Work out the finished part from the listing and answer in its coordinate system (mm). A direction names the side the tool comes from. Give positions to 0.01 mm unless a question says otherwise; leave off trailing zeros. Loops run counter-clockwise (first coordinate to the right, second up) from the corner with the lowest first, then second, coordinate; pieces in that order, holes last. Notation, with made-up numbers: M -9,-35.75 L 19,-35.75 A20 cw 19,-0.75 Z; hole C -13.75,52 d11. An arc over 180 degrees is marked long. Write item = value, one per line. Start each with the question number.
1. Section C-C on x = -25.5 is taken. Determine the outline of the cut face in (y, z) (3 decimals).
2. The mould has two halves that part along Y. Classify faces 1 (the face through (7.2, -39.1, 3.7)), 2 (the face through (14, -39, 2)), 3 (the face through (-20.855, -58.623, 23.909)): released by +Y, released by -Y, zero draft, split by the parting line, or undercut.
3. Consider L1, parallel to Y at x = 9, z = 2.15 (3 decimals); L2, parallel to X at y = -39.5, z = 3; L3, parallel to Z at x = -28, y = -44.25. Determine where each line is inside the solid, lowest interval first. Write a range as [from, to].
4. Section A-A on x = 9 is taken. Determine the outline of the cut face in (y, z) (3 decimals), plus the area to 3 significant figures.
5. Flat-ended cylindrical pins translate along their axes: pin 1 Ø2 at (y, z) = (-55, 27) entering from -X; pin 2 Ø5 at (x, z) = (-25, 22.5) entering from +Y (3 decimals); pin 3 Ø1.5 at (y, z) = (-40.5, 17.5) entering from -X; pin 4 Ø8 at (y, z) = (-44.5, 4.5) entering from +X. Find the tip coordinate at first contact, or state that the pin passes through.
6. For faces 4 (the face through (12, -38, 5)), 5 (the face through (-20, -55, 27)), 6 (the face through (-39.1, -35.38, 29.02)), 7 (the face through (-30, -55, 27)), determine the directions among +Z, -Z, +X, -X, +Y, -Y from which every point of the face is accessible in a straight line to the end or side of a thin tool.
7. Section B-B on z = 24 is taken. Determine the outline of the cut face in (x, y) (3 decimals).
8. Section D-D on z = 3 is taken. Determine the outline of the cut face in (x, y) (3 decimals), plus the area to 3 significant figures.
Autodesk Inventor part; units mm, degrees
ref_plane "РабПлоскость1" through (0, 0, 0) normal (0, 0, 1) x (1, 0, 0)
ref_plane "YZ Plane" through (0, 0, 0) normal (1, 0, 0) x (0, 1, 0)
ref_plane "XZ Plane" through (0, 0, 0) normal (0, 1, 0) x (-1, 0, 0)
ref_plane "РабПлоскость1" through (0, 0, 0) normal (0, 0, 1) x (1, 0, 0)
sketch "Эскиз1" plane through (0, 0, 0) normal (0, 0, 1) x (1, 0, 0)
  line L0 (-6, -50.525) -> (-6, 46.475)
  arc A0 (-10, -54.525) -> (-6, -50.525) centre (-10, -50.525) ccw
  line L1 (-36, -54.525) -> (-10, -54.525)
  arc A1 (-40, -50.525) -> (-36, -54.525) centre (-36, -50.525) ccw
  line L2 (-40, 46.475) -> (-40, -50.525)
  circle A2 centre (-1, -39.525) radius 5
  line L3 (5, 13.475) -> (5, 17.5589)
  line L4 (14, -44.525) -> (4, -44.525)
  line L5 (4, -44.525) -> (4, -34.525)
  line L6 (4, -34.525) -> (14, -34.525)
  line L7 (14, -34.525) -> (14, -44.525)
  line L8 (4, -44.525) -> (-1, -44.525)
  line L9 (-1, -44.525) -> (-1, -34.525)
  line L10 (-1, -34.525) -> (4, -34.525)
  line L11 (4, -34.525) -> (4, -44.525)
  point P0 (0, 0)
  dimension "d0" = 10
  dimension "d1" = 10
  dimension "d2" = 5
  dimension "d3" = 10
  dimension "d4" = 15
  dimension "d5" = 20
extrude "Выдавливание1" add sketch "Эскиз1" along normal blind 5
sketch "Эскиз2" plane through (0, 0, 5) normal (0, 0, 1) x (1, 0, 0)
  line L0 (-1, -44.525) -> (14, -44.525)
  line L1 (14, -44.525) -> (14, -34.525)
  line L2 (14, -34.525) -> (-1, -34.525)
  arc A0 (-1, -34.525) -> (-1, -44.525) centre (-1, -39.525) ccw
  circle A1 centre (-1, -39.525) radius 5
  line L3 (-1, -44.525) -> (4, -44.525)
  line L4 (4, -44.525) -> (4, -34.525)
  line L5 (4, -34.525) -> (-1, -34.525)
  line L6 (-1, -34.525) -> (-1, -44.525)
  point P0 (0, 0)
  point P1 (4, -44.525)
  dimension "d8" = 10
extrude "Выдавливание2" add sketch "Эскиз2" along normal blind 22.5 contours A1 L4 L0 | L6 A1 | A0 L6 | L2 L4 A1
sketch "Эскиз3" plane through (0, 0, 27.5) normal (0, 0, 1) x (1, 0, 0)
  line L0 (-1, -44.525) -> (4, -44.525)
  line L1 (4, -44.525) -> (4, -34.525)
  line L2 (4, -34.525) -> (-1, -34.525)
  arc A0 (-1, -34.525) -> (-1, -44.525) centre (-1, -39.525) ccw
  line L3 (4, -34.525) -> (-40, -34.525)
  line L4 (-40, -34.525) -> (-40, -44.525)
  line L5 (-40, -44.525) -> (4, -44.525)
  line L6 (4, -44.525) -> (4, -34.525)
  line L7 (-40, 46.475) -> (-40, -50.525)
  line L8 (-30, -34.525) -> (-20, -34.525)
  line L9 (-20, -34.525) -> (-20, -59.525)
  line L10 (-20, -59.525) -> (-30, -59.525)
  line L11 (-30, -59.525) -> (-30, -34.525)
  line L12 (-36, -54.525) -> (-10, -54.525)
  point P0 (0, 0)
  point P1 (-1, -34.525)
  point P2 (-20, -44.525)
  point P3 (-30, -44.525)
  dimension "d11" = 0
  dimension "d12" = 10
  dimension "d24" = 10
  dimension "d25" = 10
  dimension "d26" = 5
extrude "Выдавливание3" add sketch "Эскиз3" along normal blind 3
sketch "Эскиз4" plane through (0, 0, 5) normal (0, 0, 1) x (1, 0, 0)
  line L0 (4, -34.525) -> (4, -44.525)
  line L1 (4, -44.525) -> (14, -44.525)
  line L2 (14, -44.525) -> (14, -34.525)
  line L3 (14, -34.525) -> (4, -34.525)
  circle A0 centre (9, -39.525) radius 1.6899
  point P0 (0, 0)
hole "Отверстие1" at (9, -39.525, 5) direction (0, 0, -1) diameter 3.4 end through all countersink diameter 6.3 countersink angle 90
fillet "Сопряжение1" radius 2 2 edges at (14, -34.525, 2.5) (14, -44.525, 2.5)
fillet "Сопряжение2" radius 3 2 edges at (4, -39.525, 5) (4, -39.525, 30.5)
sketch "Эскиз5" plane through (0, 0, 27.5) normal (0, 0, -1) x (-1, 0, 0)
  line L0 (30, -59.525) -> (20, -59.525)
  line L1 (30, -44.525) -> (30, -59.525)
  line L2 (20, -59.525) -> (30, -59.525)
  line L3 (30, -59.525) -> (30, -54.525)
  line L4 (30, -54.525) -> (20, -54.525)
  line L5 (20, -54.525) -> (20, -59.525)
  point P0 (0, 0)
  dimension "d27" = 5
extrude "Выдавливание4" add sketch "Эскиз5" along normal blind 10
fillet "Сопряжение3" radius 3 8 edges at (-20, -44.525, 29) (-30, -44.525, 29) (-40, -44.525, 29) (-40, -34.525, 29) (-20, -59.525, 24) (-30, -59.525, 24) (-25, -59.525, 30.5) (-25, -59.525, 17.5)
properties part number "FrontBracket" material "Пластик ПАЭК"
Verdict:
q1.outline = M -59.525,20.5 A3 ccw -56.525,17.5 L -54.525,17.5 L -54.525,27.5 L -34.525,27.5 L -34.525,30.5 L -56.525,30.5 A3 ccw -59.525,27.5 Z
q2.face_1 = undercut
q2.face_2 = zero draft
q2.face_3 = released by -Y
q3.L1 = [-44.525, -41.225], [-37.825, -34.525]
q3.L2 = [-6, 7.3], [10.7, 14]
q3.L3 = [27.5, 30.5]
q4.outline = M -44.525,0 L -41.225,0 L -41.225,3.55 L -42.675,5 L -44.525,5 Z; M -37.825,0 L -34.525,0 L -34.525,5 L -36.375,5 L -37.825,3.55 Z
q4.area = 30.9 mm2
q5.pin_1 = -30
q5.pin_2 = -54.525
q5.pin_3 = -5.99
q5.pin_4 = 14
q6.face_4 = +Z, +X, +Y, -Y
q6.face_5 = +Z, -Z, +X, -Y
q6.face_6 = +Z, -Z, -X, +Y
q6.face_7 = +Z, -Z, -X, -Y
q7.outline = M -30,-56.525 A3 ccw -27,-59.525 L -23,-59.525 A3 ccw -20,-56.525 L -20,-54.525 L -30,-54.525 Z; M -1,-44.525 L 4,-44.525 L 4,-34.525 L -1,-34.525 A5 ccw Z
q8.outline = M -1,-44.525 L 12,-44.525 A2 ccw 14,-42.525 L 14,-36.525 A2 ccw 12,-34.525 L -1,-34.525 A5 ccw Z; hole C 9,-39.525 d3.4
q8.area = 178 mm2
